Could you check a few things on this model? Use its own coordinates, in mm. A direction names the side the tool comes from. Give positions to 0.01 mm unless a question says otherwise; leave off trailing zeros. Order: outer loops, then holes, each group sorted by start corner. A loop starts at its lowest first (then second) coordinate and runs counter-clockwise, first axis right, second up. Notation, with made-up numbers: (-6.75, 23) -> (35.25, 23) arc R14 ccw to (35.25, 48) -> close; hole circle Ø3 at (40.5, 51.5). An arc over 180 degrees is marked (long way). Write each question's results on one line, items separated by ' | '.
```python
from build123d import *

# Parameters (mm, degrees)
F0_R     = 3.175
F1_DEPTH = 3.175


with BuildPart() as f1:
    # F0 (on Top) → F1 (new body)
    with BuildSketch(Plane.XY):
        Polygon((140.5679399306, 1060.2679701805), (115.9471851349, 1045.4435404041), (312.7971851349, 926.9179701805), (312.7971851349, 956.5668297334), align=None)
        with Locations((300.0971851349, 945.9679701805)):
            Circle(F0_R, mode=Mode.SUBTRACT)
        Polygon((115.9471851349, 1075.092399957), (140.5679399306, 1060.2679701805), (312.7971851349, 1163.9691106276), (312.7971851349, 1193.6179701805), align=None)
        with Locations((300.0971851349, 1174.5679701805)):
            Circle(F0_R, mode=Mode.SUBTRACT)
        Polygon((-80.9028148651, 956.5668297334), (-80.9028148651, 926.9179701805), (115.9471851349, 1045.4435404041), (91.3264303392, 1060.2679701805), align=None)
        with Locations((-68.2028148651, 945.9679701805)):
            Circle(F0_R, mode=Mode.SUBTRACT)
        Polygon((-80.9028148651, 1193.6179701805), (-80.9028148651, 1163.9691106276), (91.3264303392, 1060.2679701805), (115.9471851349, 1075.092399957), align=None)
        with Locations((-68.2028148651, 1174.5679701805)):
            Circle(F0_R, mode=Mode.SUBTRACT)
        Polygon((91.3264303392, 1060.2679701805), (115.9471851349, 1045.4435404041), (140.5679399306, 1060.2679701805), (115.9471851349, 1075.092399957), align=None)
    extrude(amount=F1_DEPTH)


solid = f1.part
```
Q1. I'm going to push flat-ended pins straight in: pin 1 Ø5 at (x, y) = (300.1, 945.97) entering from +Z; pin 2 Ø1 at (x, z) = (258, 1) entering from -Y. Where does each tip first touch, or does it pass through?
Here are the results:
pin 1: passes through | pin 2: stops at y = 959.61
Q2. Thinking about a two-plate mould opening in X: for faces 1 (the flat face through (115, 1061, 0)), 2 (the flat face through (18.9, 1133.526, 1.565)), 3 (the flat face through (4.01, 1112.84, 1.57)), 4 (the flat face through (16.14, 985.35, 1.57)), which applies, +X half, -X half, draft (parallel to the pull), parting line (faces both ways), or undercut?
Here are the results:
face 1: draft | face 2: undercut | face 3: -X half | face 4: undercut
Q3. I need wall thicknesses on line 1 along X through (y, z) = (1007.5, 2.5); line 2 along X through (y, z) = (1150.5, 0.9); line 3 along Y through (x, z) = (-21, 1.5). Which ranges of each line are inside material? Lowest first, please.
Here are the results:
line 1: x = 3.69 to 52.93, 178.96 to 228.21 | line 2: x = -58.53 to -9.29, 241.19 to 290.43 | line 3: y = 962.99 to 992.63, 1127.9 to 1157.55
Q4. For faces 5 (the flat face through (215.75, 1135.185, 1.565)), 6 (the flat face through (212.994, 987.01, 1.565)), 7 (the flat face through (6.417, 1009.143, 1.565)), 8 (the flat face through (227.89, 1007.69, 1.57)), which set-ups out of +Z, -Z, +X, -X, +Y, -Y let a thin tool reach every point of the face, with its end or its side?
Here are the results:
face 5: +Z, -Z, +Y | face 6: +Z, -Z, -Y | face 7: +Z, -Z, -X | face 8: +Z, -Z, +X
Q5. Suppose I cut it at A-A on y = 1135. Please give me the cut outline in (x, z) (3 decimals).
Here are the results:
outline: (-32.79, 0) -> (16.451, 0) -> (16.451, 3.175) -> (-32.79, 3.175) -> close; (215.443, 0) -> (264.685, 0) -> (264.685, 3.175) -> (215.443, 3.175) -> close
Q6. Suppose I cut it at B-B on x = 198.5. Please give me the cut outline in (y, z) (1 decimal), and give its area (3 significant figures).
Here are the results:
outline: (995.7, 0) -> (1025.4, 0) -> (1025.4, 3.2) -> (995.7, 3.2) -> close; (1095.1, 0) -> (1124.8, 0) -> (1124.8, 3.2) -> (1095.1, 3.2) -> close | area: 188 mm²
Q7. Suppose I cut it at C-C on z = 1.35. Please give me the cut outline in (x, y) (3 decimals), and give its area (3 significant figures).
Here are the results:
outline: (-80.903, 926.918) -> (115.947, 1045.444) -> (312.797, 926.918) -> (312.797, 956.567) -> (140.568, 1060.268) -> (312.797, 1163.969) -> (312.797, 1193.618) -> (115.947, 1075.092) -> (-80.903, 1193.618) -> (-80.903, 1163.969) -> (91.326, 1060.268) -> (-80.903, 956.567) -> close; hole circle Ø6.35 at (-68.203, 945.968); hole circle Ø6.35 at (-68.203, 1174.568); hole circle Ø6.35 at (300.097, 945.968); hole circle Ø6.35 at (300.097, 1174.568) | area: 22,500 mm²
Q8. Suppose I cut it at D-D on y = 1050. Please give me the cut outline in (x, z) (3 decimals).
Here are the results:
outline: (74.273, 0) -> (157.621, 0) -> (157.621, 3.175) -> (74.273, 3.175) -> close
